Work out the finished part from the listing and answer in its coordinate system (mm). A direction names the side the tool comes from. Round coordinates to 2 decimals unless told otherwise and drop trailing zeros. Order: outer loops, then holes, each group sorted by start corner. A loop starts at its lowest first (then second) coordinate and runs counter-clockwise, first axis right, second up. Notation, with made-up numbers: M 34,77 L 48,77 A24 ccw 48,99 Z; hole C 82.25,77.5 d1. An arc over 180 degrees is marked long. Answer as a JSON object with one key per item and string values. Group by question number.
from build123d import *

# Parameters (mm, degrees)
SKETCH_1_W          = 10
SKETCH_1_H          = 10
SKETCH_1_W_2        = 8
SKETCH_1_H_2        = 8
EXTRUDE_1_DEPTH     = 187.2
SKETCH_2_R          = 2
CUT_EXTRUDE_1_DEPTH = 188.533570328


with BuildPart() as part:
    # ｽｹｯﾁ1 → 押し出し-薄板1 (new body)
    with BuildSketch(Plane(origin=(0, 0, 0), x_dir=(0, 0, -1), z_dir=(1, 0, 0))):
        Rectangle(SKETCH_1_W, SKETCH_1_H)
        Rectangle(SKETCH_1_W_2, SKETCH_1_H_2, mode=Mode.SUBTRACT)
    extrude(amount=EXTRUDE_1_DEPTH)

    # ｽｹｯﾁ2 → ｶｯﾄ - 押し出し1 (cut, through all)
    with BuildSketch(Plane.XY.offset(5)):
        with Locations((7.5, 0)):
            Circle(SKETCH_2_R)
        with Locations(Location((179.7, 0, 0), (0, 0, 180))):
            Circle(SKETCH_2_R)
    extrude(amount=-CUT_EXTRUDE_1_DEPTH, mode=Mode.SUBTRACT)


solid = part.part
Item 1: Consider L1, parallel to Z at x = 96, y = -2; L2, parallel to Y at x = 7.5, z = -4.65. Determine where each line is inside the solid, lowest interval first.
Item 2: Find section D-D (x = 92.5). Give the vertices of the cut face in (y, z), and give its area (3 significant figures).
Item 3: The mould has two halves that part along Y. Classify faces 1 (the flat face through (187.2, 0.1, 4.5)), 2 (the cylindrical face through (5.502, 0.088, 4.507)), 3 (the flat face through (92, 0, 4)), 4 (the flat face through (92, 5, 0)): +Y half, -Y half, draft (parallel to the pull), parting line (faces both ways), or undercut.
Item 4: A tool of negligible diameter and unlimited length cuts with its end or side. For faces 5 (the flat face through (0, 0.1, 4.5)), 6 (the flat face through (92, 0, -4)), from which of +Z, -Z, +X, -X, +Y, -Y can it reach the whole face along a straight path? Write none if from no direction.
Item 5: Find section C-C (y = 0). Give the vertices of the cut face in (x, z).
Item 6: Find section A-A (x = 179.7). Give the vertices of the cut face in (y, z), and give its area (3 significant figures).
Item 7: Find section B-B (z = 2). Give the vertices of the cut face in (x, y).
Responses:
{
 "1": {"L1": "z = -5 to -4, 4 to 5", "L2": "y = -5 to -2, 2 to 5"},
 "2": {"outline": "M -5,-5 L 5,-5 L 5,5 L -5,5 Z; hole M -4,-4 L 4,-4 L 4,4 L -4,4 Z", "area": "36.0 mm^2"},
 "3": {"face 1": "draft", "face 2": "undercut", "face 3": "undercut", "face 4": "+Y half"},
 "4": {"face 5": "+Z, -Z, -X, +Y, -Y", "face 6": "+X, -X"},
 "5": {"outline": "M 0,-5 L 5.5,-5 L 5.5,-4 L 0,-4 Z; M 0,4 L 5.5,4 L 5.5,5 L 0,5 Z; M 9.5,-5 L 177.7,-5 L 177.7,-4 L 9.5,-4 Z; M 9.5,4 L 177.7,4 L 177.7,5 L 9.5,5 Z; M 181.7,-5 L 187.2,-5 L 187.2,-4 L 181.7,-4 Z; M 181.7,4 L 187.2,4 L 187.2,5 L 181.7,5 Z"},
 "6": {"outline": "M -5,-5 L -2,-5 L -2,-4 L -4,-4 L -4,4 L -2,4 L -2,5 L -5,5 Z; M 2,-5 L 5,-5 L 5,5 L 2,5 L 2,4 L 4,4 L 4,-4 L 2,-4 Z", "area": "28.0 mm^2"},
 "7": {"outline": "M 0,-5 L 187.2,-5 L 187.2,-4 L 0,-4 Z; M 0,4 L 187.2,4 L 187.2,5 L 0,5 Z"}
}
